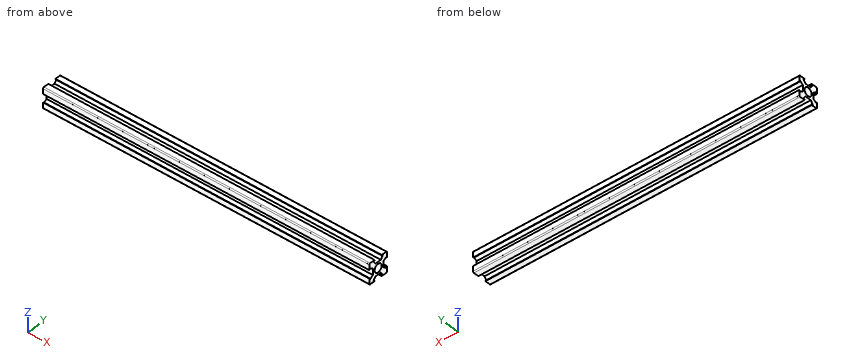
from build123d import *

# Parameters (mm, degrees)
SKETCH_1_W                       = 321
SKETCH_1_H                       = 10
EXTRUDE_1_DEPTH                  = 10
SKETCH_2_R                       = 4
CUT_EXTRUDE_1_DEPTH              = 1270
CUT_EXTRUDE_2_DEPTH              = 1270
FILLET_1_R                       = 1
PATTERN_CIRCULAR_2_COUNT         = 4
FILLET_1_OF_PATTERN_CIRCULAR_2_R = 1


with BuildPart() as part:
    # 草图1 → 凸台-拉伸1 (new body)
    with BuildSketch(Plane.XY):
        with Locations((93.981285353, -6.397869645)):
            Rectangle(SKETCH_1_W, SKETCH_1_H)
    extrude_1 = extrude(amount=EXTRUDE_1_DEPTH)

    # 草图2 → 切除-拉伸1 (cut)
    with BuildSketch(Plane(origin=(254.481285353, 0, 0), x_dir=(0, 0, -1), z_dir=(1, 0, 0))):
        with Locations((0, -11.397869645)):
            Circle(SKETCH_2_R)
    cut_extrude_1 = extrude(amount=-CUT_EXTRUDE_1_DEPTH, mode=Mode.SUBTRACT)

    # 草图3 → 切除-拉伸2 (cut)
    with BuildSketch(Plane(origin=(254.481285353, 0, 0), x_dir=(0, 0, -1), z_dir=(1, 0, 0))):
        Polygon((-4, -1.397869645), (0, -1.397869645), (0, -5.397869645), (-3, -5.397869645), (-5.5, -1.897869645), (-4, -1.897869645), align=None)
        Polygon((-10, -7.397869645), (-10, -11.397869645), (-6, -11.397869645), (-6, -8.397869645), (-9.5, -5.897869645), (-9.5, -7.397869645), align=None)
    cut_extrude_2 = extrude(amount=-CUT_EXTRUDE_2_DEPTH, mode=Mode.SUBTRACT)

    # 圆角1
    fillet_1_edges = [part.edges().sort_by_distance(p)[0] for p in [
        (93.981285353, -1.397869645, 10),
    ]]
    fillet(fillet_1_edges, radius=FILLET_1_R)

    # 阵列(圆周)2: 凸台-拉伸1, 切除-拉伸1, 切除-拉伸2 ×4 about axis
    pattern_circular_2_axis = Axis((0, -11.397869645, 0), (1, 0, 0))
    add([extrude_1.rotate(pattern_circular_2_axis, i * 360 / PATTERN_CIRCULAR_2_COUNT) for i in range(1, PATTERN_CIRCULAR_2_COUNT)])
    add([cut_extrude_1.rotate(pattern_circular_2_axis, i * 360 / PATTERN_CIRCULAR_2_COUNT) for i in range(1, PATTERN_CIRCULAR_2_COUNT)], mode=Mode.SUBTRACT)
    add([cut_extrude_2.rotate(pattern_circular_2_axis, i * 360 / PATTERN_CIRCULAR_2_COUNT) for i in range(1, PATTERN_CIRCULAR_2_COUNT)], mode=Mode.SUBTRACT)

    # 圆角1 of 阵列(圆周)2
    fillet_1_of_pattern_circular_2_edges = [part.edges().sort_by_distance(p)[0] for p in [
        (93.981285353, -21.397869645, 10),
        (93.981285353, -21.397869645, -10),
        (93.981285353, -1.397869645, -10),
    ]]
    fillet(fillet_1_of_pattern_circular_2_edges, radius=FILLET_1_OF_PATTERN_CIRCULAR_2_R)


solid = part.part
Build history of the part. All positions in model axes, mm. Give positions to 0.01 mm unless a question says otherwise; leave off trailing zeros. Order: outer loops, then holes, each group sorted by start corner. A loop starts at its lowest first (then second) coordinate and runs counter-clockwise, first axis right, second up. Notation, with made-up numbers: M 22.25,75 L 79.25,75 A17 ccw 79.25,93 Z; hole C -39,28 d8. An arc over 180 degrees is marked long. Put each result on its own line as item: value.
Item 1: Cut at A-A on z = 0. Write the cut outline in (x, y).
Results are:
outline: M -66.52,-17.4 L 254.48,-17.4 L 254.48,-15.4 L -66.52,-15.4 Z; M -66.52,-7.4 L 254.48,-7.4 L 254.48,-5.4 L -66.52,-5.4 Z
Item 2: Drop flat-ended pins along their axis: pin 1 Ø0.6 at (x, y) = (152, -21) entering from +Z; pin 2 Ø0.6 at (x, z) = (128.5, -10) entering from +Y; pin 3 Ø0.6 at (x, z) = (96.5, 10) entering from -Y. Give the stop position or say it passes through.
Results are:
pin 1: z = 9.95
pin 2: y = -1.68
pin 3: y = -21.11
Item 3: Wall check: probe 1 along Z at (x, y) = (114, -16.5); probe 2 along Y at (x, z) = (61.5, -0.5); probe 3 along Z at (x, y) = (-50.5, -18.75). Give the ranges that are in metal, low to high.
Results are:
probe 1: -10 to -9.5, -8.94 to 8.94, 9.5 to 10
probe 2: -17.4 to -15.37, -7.43 to -5.4
probe 3: -10 to -3.97, 3.97 to 10
